Source: CAD feature listing. Evaluate the final solid. Frame: model axes, mm. A direction names the side the tool comes from. Give positions to 0.01 mm unless a question says otherwise; leave off trailing zeros. Order: outer loops, then holes, each group sorted by start corner. A loop starts at its lowest first (then second) coordinate and runs counter-clockwise, first axis right, second up. Notation, with made-up numbers: (5.5, -39.5) -> (37.5, -39.5) arc R23 ccw to (37.5, -18.5) -> close; hole circle Ø4 at (-25.5, -35.75). An arc over 180 degrees is marked (long way). Use one line per item in the form item = value. Start each with the question number.
from build123d import *

# Parameters (mm, degrees)
SKETCH_1_W      = 100
SKETCH_1_H      = 60
EXTRUDE_1_DEPTH = 50
SHELL_1_T       = -5


with BuildPart() as part:
    # 草图1 → 凸台-拉伸1 (new body)
    with BuildSketch(Plane.XY):
        Rectangle(SKETCH_1_W, SKETCH_1_H)
    extrude(amount=EXTRUDE_1_DEPTH)

    # 抽壳1
    shell_1_openings = [part.faces().sort_by_distance(p)[0] for p in [
        (0, 0, 50),
    ]]
    offset(amount=SHELL_1_T, openings=shell_1_openings, kind=Kind.INTERSECTION)


solid = part.part
1) Material intervals for probe 1 along X at (y, z) = (11, 39.5); probe 2 along Y at (x, z) = (-10, 31.5); probe 3 along Z at (x, y) = (-33, -11), sorted ascending.
2) Cut plane B-B, the plane x = -43.5. Return the cut outline in (y, z), plus the area to 3 significant figures.
3) Cut plane A-A, the plane z = 21. Return the cut outline in (x, y), plus the area to 3 significant figures.
4) Reachability of faces 1 (the face through (-1, 0, 0)), 2 (the face through (-1, 0, 5)) from +Z, -Z, +X, -X, +Y, -Y: full face, straight path, thin tool, end or side. Return the list, or none.
5) Pin query (flat end, axial travel): pin 1 (12 mm diameter, centred on x = -25, y = 18.5, fed in from +Z). Return the tip coordinate at first contact, or that it passes through.
6) Cut plane C-C, the plane y = -14.5. Return the cut outline in (x, z), plus the area to 3 significant figures.
7) Draft query along Y for faces 3 (the face through (50, 0, 25)), 4 (the face through (-1, 30, 25)), 5 (the face through (-45, 0, 27)). Return one class per face: +Y half, -Y half, draft (parallel to the pull), parting line (faces both ways), or undercut.
Output values:
q1.probe_1 = -50 to -45, 45 to 50
q1.probe_2 = -30 to -25, 25 to 30
q1.probe_3 = 0 to 5
q2.outline = (-30, 0) -> (30, 0) -> (30, 50) -> (25, 50) -> (25, 5) -> (-25, 5) -> (-25, 50) -> (-30, 50) -> close
q2.area = 750 mm^2
q3.outline = (-50, -30) -> (50, -30) -> (50, 30) -> (-50, 30) -> close; hole (-45, -25) -> (45, -25) -> (45, 25) -> (-45, 25) -> close
q3.area = 1,500 mm^2
q4.face_1 = -Z, +X, -X, +Y, -Y
q4.face_2 = +Z
q5.pin_1 = 5
q6.outline = (-50, 0) -> (50, 0) -> (50, 50) -> (45, 50) -> (45, 5) -> (-45, 5) -> (-45, 50) -> (-50, 50) -> close
q6.area = 950 mm^2
q7.face_3 = draft
q7.face_4 = +Y half
q7.face_5 = undercut
